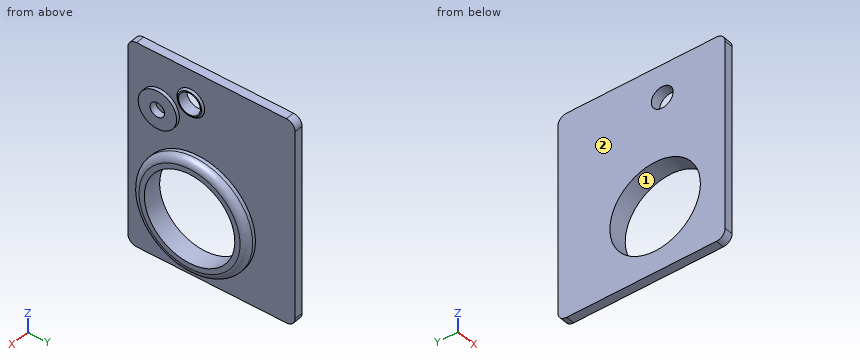
from build123d import *

# Parameters (mm, degrees)
SKETCH1_W           = 118.7383283
SKETCH1_H           = 95.637293174
SKETCH1_R           = 7.894829417
SKETCH1_R_2         = 10.963118073
SKETCH1_R_3         = 32.887608347
BOSS_EXTRUDE1_DEPTH = 5
SKETCH1_3_R         = 32.887608347
SKETCH1_3_R_2       = 25.869040911
BOSS_EXTRUDE2_DEPTH = 11
FILLET1_R           = 4
SKETCH1_4_R         = 10.963118073
SKETCH1_4_R_2       = 4.130606261
BOSS_EXTRUDE3_DEPTH = 7
SKETCH1_5_R         = 7.894829417
SKETCH1_5_R_2       = 6.243605875
BOSS_EXTRUDE4_DEPTH = 6
CHAMFER1_SIZE       = 1
FILLET2_R           = 5
SKETCH1_6_R         = 4.130606261
BOSS_EXTRUDE5_DEPTH = 3


with BuildPart() as part:
    # Sketch1 → Boss-Extrude1 (new body)
    with BuildSketch(Plane(origin=(0, 0, 0), x_dir=(0, 0, -1), z_dir=(1, 0, 0))):
        Rectangle(SKETCH1_W, SKETCH1_H)
        with Locations((-40.363308429, -11.826050305)):
            Circle(SKETCH1_R, mode=Mode.SUBTRACT)
        with Locations((-28.513672981, -29.366301206)):
            Circle(SKETCH1_R_2, mode=Mode.SUBTRACT)
        with Locations((21.052704773, -7.782501182)):
            Circle(SKETCH1_R_3, mode=Mode.SUBTRACT)
    extrude(amount=BOSS_EXTRUDE1_DEPTH)

    # Sketch1<3> → Boss-Extrude2 (add)
    with BuildSketch(Plane(origin=(0, 0, 0), x_dir=(0, 0, -1), z_dir=(1, 0, 0))):
        with Locations((21.052704773, -7.782501182)):
            Circle(SKETCH1_3_R)
        with Locations((21.052704773, -7.782501182)):
            Circle(SKETCH1_3_R_2, mode=Mode.SUBTRACT)
    extrude(amount=BOSS_EXTRUDE2_DEPTH)

    # Fillet1
    fillet1_edges = [part.edges().sort_by_distance(p)[0] for p in [
        (11, -7.782501182, 11.834903573),
    ]]
    fillet(fillet1_edges, radius=FILLET1_R)

    # Sketch1<4> → Boss-Extrude3 (add)
    with BuildSketch(Plane(origin=(0, 0, 0), x_dir=(0, 0, -1), z_dir=(1, 0, 0))):
        with Locations((-28.513672981, -29.366301206)):
            Circle(SKETCH1_4_R)
        with Locations((-28.513672981, -29.366301206)):
            Circle(SKETCH1_4_R_2, mode=Mode.SUBTRACT)
    extrude(amount=BOSS_EXTRUDE3_DEPTH)

    # Sketch1<5> → Boss-Extrude4 (add)
    with BuildSketch(Plane(origin=(0, 0, 0), x_dir=(0, 0, -1), z_dir=(1, 0, 0))):
        with Locations((-40.363308429, -11.826050305)):
            Circle(SKETCH1_5_R)
        with Locations((-40.363308429, -11.826050305)):
            Circle(SKETCH1_5_R_2, mode=Mode.SUBTRACT)
    extrude(amount=BOSS_EXTRUDE4_DEPTH)

    # Chamfer1
    chamfer1_edges = [part.edges().sort_by_distance(p)[0] for p in [
        (6, -11.826050305, 48.258137847),
    ]]
    chamfer(chamfer1_edges, length=CHAMFER1_SIZE - 0.0001)  # a hair under: the kernel refuses the full size

    # Fillet2
    fillet2_edges = [part.edges().sort_by_distance(p)[0] for p in [
        (2.5, -47.818646587, 59.36916415),
        (2.5, 47.818646587, 59.36916415),
        (2.5, 47.818646587, -59.36916415),
        (2.5, -47.818646587, -59.36916415),
    ]]
    fillet(fillet2_edges, radius=FILLET2_R)

    # Sketch1<6> → Boss-Extrude5 (add)
    with BuildSketch(Plane(origin=(0, 0, 0), x_dir=(0, 0, -1), z_dir=(1, 0, 0))):
        with Locations((-28.513672981, -29.366301206)):
            Circle(SKETCH1_6_R)
    extrude(amount=BOSS_EXTRUDE5_DEPTH)


solid = part.part
CAD build for the part. Positions are in the model's coordinates, mm. Face numbers are marked on the shaded views. Coordinates: 2 decimals unless noted, no trailing zeros. Loops run counter-clockwise (first coordinate to the right, second up) from the corner with the lowest first, then second, coordinate; pieces in that order, holes last. Notation, with made-up numbers: (73.25, -28) - (107.25, -28) arc R32 cw to (107.25, -2) - close; hole circle Ø6 at (49, 42). An arc over 180 degrees is marked (long way). Write item = value, one per line. Start each with the question number.
Q1. Cut at B-B, the plane y = 36. List the corners of the cut face in (x, z).
Q2. Cut at A-A, the plane x = 1.25. List the corners of the cut face in (y, z).
Q3. Drill centre lines: L1, parallel to X at y = -36.5, z = -4; L2, parallel to Y at x = 8.25, z = -16.5; L3, parallel to Z at x = 9.75, y = -18. Where is each one in solid material? Low to high.
Q4. Cut at C-C, the plane x = 8.75. List the corners of the cut face in (y, z).
Q5. Flat gauge pins, fed straight in: pin 1 Ø7 at (y, z) = (-14, 37.5) entering from +X; pin 2 Ø2.5 at (y, z) = (-28.5, 26.5) entering from +X; pin 3 Ø6.5 at (y, z) = (-27.5, 24) entering from +X. Where does each tip first touch, or does it go through?
Q6. Pull direction Z, two halves, no side cores. Call the marked faces 1 and 2: pulls with the +Z half, pulls with the -Z half, needs draft (parallel to the pull), parting line crosses it, or undercut.
Computed:
q1.outline = (0, -59.37) - (5, -59.37) - (5, 59.37) - (0, 59.37) - close
q2.outline = (-47.82, -54.37) arc R5 ccw to (-42.82, -59.37) - (42.82, -59.37) arc R5 ccw to (47.82, -54.37) - (47.82, 54.37) arc R5 ccw to (42.82, 59.37) - (-42.82, 59.37) arc R5 ccw to (-47.82, 54.37) - close; hole circle Ø51.74 at (-7.78, -21.05); hole circle Ø12.49 at (-11.83, 40.36)
q3.L1 = 0 to 5
q3.L2 = -40.15 to -33.25, 17.68 to 24.59
q3.L3 = -51.16 to -44.82, 2.71 to 9.05
q4.outline = circle Ø64.97 at (-7.78, -21.05); hole circle Ø51.74 at (-7.78, -21.05)
q5.pin_1 = 6
q5.pin_2 = 3
q5.pin_3 = 7
q6.face_1 = undercut
q6.face_2 = needs draft
